Check sheet for the modelled part. Datum: model origin and axes. Units: mm. Round coordinates to 2 decimals unless told otherwise and drop trailing zeros. Order: outer loops, then holes, each group sorted by start corner. A loop starts at its lowest first (then second) coordinate and runs counter-clockwise, first axis right, second up.
(1) Thickness scan on probe 1 along X at (y, z) = (-61, 2.6); probe 2 along X at (y, z) = (43, 2.3). Record the ranges inside material, lowest first.
(2) Sectioned sample at C-C, the plane x = -102. Enter the section's corners in (y, z).
(3) Sectioned sample at A-A, the plane z = 1.75. Enter the section's corners in (x, y).
(4) Sectioned sample at B-B, the plane y = -49. Enter the section's corners in (x, z).
```python
from build123d import *

# Parameters (mm, degrees)
SKETCH1_W           = 250
SKETCH1_H           = 150
BOSS_EXTRUDE1_DEPTH = 3
CHAMFER3_SIZE       = 35


with BuildPart() as part:
    # Sketch1 → Boss-Extrude1 (new body)
    with BuildSketch(Plane.XY):
        Rectangle(SKETCH1_W, SKETCH1_H)
    extrude(amount=BOSS_EXTRUDE1_DEPTH)

    # Chamfer3
    chamfer3_edges = [part.edges().sort_by_distance(p)[0] for p in [
        (-125, -75, 1.5),
        (-125, 75, 1.5),
    ]]
    chamfer(chamfer3_edges, length=CHAMFER3_SIZE)


solid = part.part
```
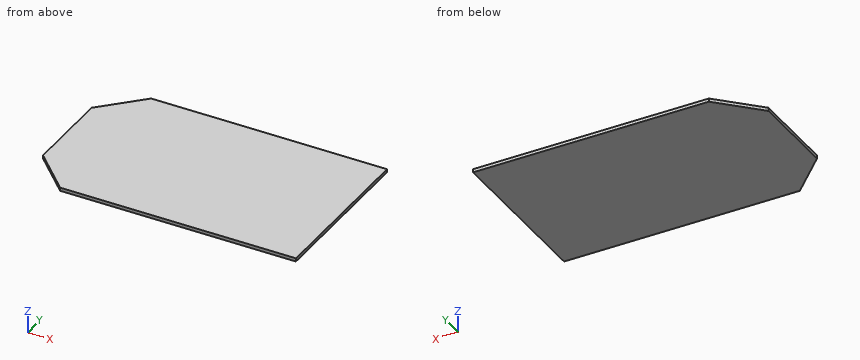
Derived:
1. probe 1: x = -104 to 125
1. probe 2: x = -122 to 125
2. outline: (-63, 0) - (63, 0) - (63, 3) - (-63, 3) - close
3. outline: (-125, -40) - (-90, -75) - (125, -75) - (125, 75) - (-90, 75) - (-125, 40) - close
4. outline: (-116, 0) - (125, 0) - (125, 3) - (-116, 3) - close
